from build123d import *

# Parameters (mm, degrees)
SKETCH_1_R               = 4
EXTRUDE_1_DEPTH          = 20
SKETCH_2_W               = 14
SKETCH_2_H               = 7
SKETCH_2_W_2             = 3.5
SKETCH_2_H_2             = 4
CUT_EXTRUDE_1_DEPTH      = 39.890872965
FILLET_1_R               = 2
FILLET_2_R               = 2
FILLET_4_R               = 1
CUT_EXTRUDE_2_DEPTH      = 42.003048667
CUT_EXTRUDE_2_DEPTH_BACK = 42.003048667
SKETCH_4_R               = 1.5
SKETCH_5_W               = 4.377501001
SKETCH_5_H               = 5
CUT_EXTRUDE_3_DEPTH      = 39.890873036


with BuildPart() as part:
    # 草图1 → 凸台-拉伸1 (new body)
    with BuildSketch(Plane.XY):
        Polygon((-25, 7.5), (25, 7.5), (32.5, 7.5), (32.5, -7.5), (25, -7.5), (-25, -7.5), (-32.5, -7.5), (-32.5, 7.5), align=None)
        with Locations((-25, 0)):
            Circle(SKETCH_1_R, mode=Mode.SUBTRACT)
        with Locations((25, 0)):
            Circle(SKETCH_1_R, mode=Mode.SUBTRACT)
    extrude(amount=EXTRUDE_1_DEPTH)

    # 草图2 → 切除-拉伸1 (cut, through all)
    with BuildSketch(Plane.XY.offset(20)):
        with Locations((-11, 0)):
            Rectangle(SKETCH_2_W, SKETCH_2_H)
        with Locations((11, 0)):
            Rectangle(SKETCH_2_W, SKETCH_2_H)
        with Locations((0, 5.5)):
            Rectangle(SKETCH_2_W_2, SKETCH_2_H_2)
        with Locations((0, -5.5)):
            Rectangle(SKETCH_2_W_2, SKETCH_2_H_2)
    extrude(amount=-CUT_EXTRUDE_1_DEPTH, mode=Mode.SUBTRACT)

    # 圆角1
    fillet_1_edges = [part.edges().sort_by_distance(p)[0] for p in [
        (-1.75, 7.5, 10),
        (1.75, 7.5, 10),
        (-1.75, -7.5, 10),
        (1.75, -7.5, 10),
    ]]
    fillet(fillet_1_edges, radius=FILLET_1_R)

    # 圆角2
    fillet_2_edges = [part.edges().sort_by_distance(p)[0] for p in [
        (-4, 3.5, 10),
        (-4, -3.5, 10),
        (-18, -3.5, 10),
        (-18, 3.5, 10),
        (18, 3.5, 10),
        (18, -3.5, 10),
        (4, -3.5, 10),
        (4, 3.5, 10),
    ]]
    fillet(fillet_2_edges, radius=FILLET_2_R)

    # 圆角4
    fillet_4_edges = [part.edges().sort_by_distance(p)[0] for p in [
        (-1.75, 3.5, 10),
        (1.75, 3.5, 10),
        (-1.75, -3.5, 10),
        (1.75, -3.5, 10),
    ]]
    fillet(fillet_4_edges, radius=FILLET_4_R)

    # 草图4 → 切除-拉伸2 (cut, two sides: drawn at the far end of the back side and taken through both)
    with BuildSketch(Plane(origin=(0, 7.5, 0), x_dir=(1, 0, 0), z_dir=(0, 1, 0)).offset(-CUT_EXTRUDE_2_DEPTH_BACK)):
        with Locations(Location((-25, -10, 0), (0, 0, 180))):
            Circle(SKETCH_4_R)
        with Locations(Location((25, -10, 0), (0, 0, 180))):
            Circle(SKETCH_4_R)
    extrude(amount=CUT_EXTRUDE_2_DEPTH + CUT_EXTRUDE_2_DEPTH_BACK, mode=Mode.SUBTRACT)

    # 草图5 → 切除-拉伸3 (cut, through all)
    with BuildSketch(Plane.XY.offset(20)):
        with Locations((-30.3112495, 0)):
            Rectangle(SKETCH_5_W, SKETCH_5_H)
        with Locations((30.3112495, 0)):
            Rectangle(SKETCH_5_W, SKETCH_5_H)
    extrude(amount=-CUT_EXTRUDE_3_DEPTH, mode=Mode.SUBTRACT)


solid = part.part
Read the model definition and answer for the solid it produces. Units are mm, in the model's axes. A direction names the side the tool comes from. Coordinates: 2 decimals unless noted, no trailing zeros. Loops run counter-clockwise (first coordinate to the right, second up) from the corner with the lowest first, then second, coordinate; pieces in that order, holes last.
Q1. Each of these flat-tipped pins is pushed along its axis until it touches: pin 1 Ø2 at (x, z) = (0, 12) entering from -Y; pin 2 Ø2 at (x, z) = (-2.5, 9.5) entering from -Y; pin 3 Ø2.5 at (y, z) = (-0.5, 6.5) entering from +X. Where does it stop, or does it pass through?
Q2. The part is cut by section B-B on x = 17. Write down the section's boundary in (y, z).
Q3. The mould has two halves that part along Z. Classify faces 6 (the face through (-26.386, -5.63, 9.425)), 7 (the face through (-2.32, 6.9, 9.86)): +Z half, -Z half, draft (parallel to the pull), parting line (faces both ways), or undercut.
Q4. The part is cut by section A-A on x = 25. Write down the section's boundary in (y, z), and give its area (3 significant figures).
Q5. Consider probe 1 along X at (y, z) = (4.85, 10); probe 2 along X at (y, z) = (0, 7.5). Determine where each line is inside the solid, lowest interval first.
Q6. The part is cut by section C-C on z = 10. Give the number of separate pieces and of enclosed holes in the cut face, and give its area (3 significant figures).
Q7. Which of the six approach directions +Z, -Z, +X, -X, +Y, -Y give full straight-line access (tool end or side, diameter ignored) to faces 1 (the face through (-11, 3.5, 10)), 2 (the face through (2.35, 6.93, 9.86)), 3 (the face through (-2.35, -6.93, 9.86)), 4 (the face through (-30, -2.5, 10)), 5 (the face through (30, 2.5, 10))?
Results below:
1. pin 1: stops at y = -3.53
1. pin 2: stops at y = -7.48
1. pin 3: stops at x = 21.4
2. outline: (-7.5, 0) - (-3.23, 0) - (-3.23, 20) - (-7.5, 20) - close; (3.23, 0) - (7.5, 0) - (7.5, 20) - (3.23, 20) - close
3. face 6: undercut
3. face 7: draft
4. outline: (-7.5, 0) - (-4, 0) - (-4, 8.5) - (-7.5, 8.5) - close; (-7.5, 11.5) - (-4, 11.5) - (-4, 20) - (-7.5, 20) - close; (4, 0) - (7.5, 0) - (7.5, 8.5) - (4, 8.5) - close; (4, 11.5) - (7.5, 11.5) - (7.5, 20) - (4, 20) - close
4. area: 119 mm2
5. probe 1: x = -32.5 to -26.5, -23.5 to -1.75, 1.75 to 23.5, 26.5 to 32.5
5. probe 2: x = -21 to -18, -4 to 4, 18 to 21
6. separate pieces: 5
6. enclosed holes: 2
6. area: 574 mm2
7. face 1: +Z, -Z
7. face 2: +Z, -Z, +Y
7. face 3: +Z, -Z, -Y
7. face 4: +Z, -Z, -X
7. face 5: +Z, -Z, +X
